Autodesk Inventor part; units mm, degrees
ref_plane "YZ Plane" through (0, 0, 0) normal (1, 0, 0) x (0, 1, 0)
ref_plane "XZ Plane" through (0, 0, 0) normal (0, 1, 0) x (-1, 0, 0)
ref_plane "XY Plane" through (0, 0, 0) normal (0, 0, 1) x (1, 0, 0)
ref_plane "Work Plane1" through (0, -18, -3) normal (1, 0, 0) x (0, 0, -1)
sketch "Sketch2" plane through (0, -18, -3) normal (1, 0, 0) x (0, 0, -1)
  line L0 (-2.3324, 4.2554) -> (0, 4.2554)
  arc A0 (-3, 4) -> (-2.3324, 4.2554) centre (-3, 5) ccw
  line L1 (-3, 0.5) -> (-3, 4)
  line L2 (0, 0.5) -> (-3, 0.5)
  line L3 (0, 4.2554) -> (0, 0.5)
  line L4 (0, 15.7446) -> (-2.3324, 15.7446)
  line L5 (0, 19.5) -> (0, 15.7446)
  line L6 (-3, 19.5) -> (0, 19.5)
  line L7 (-3, 16) -> (-3, 19.5)
  arc A1 (-2.3324, 15.7446) -> (-3, 16) centre (-3, 15) ccw
  line L8 (20, 4.2554) -> (22.3324, 4.2554)
  line L9 (20, 0.5) -> (20, 4.2554)
  line L10 (23, 0.5) -> (20, 0.5)
  line L11 (23, 4) -> (23, 0.5)
  arc A2 (22.3324, 4.2554) -> (23, 4) centre (23, 5) ccw
  line L12 (22.3324, 15.7446) -> (20, 15.7446)
  arc A3 (23, 16) -> (22.3324, 15.7446) centre (23, 15) ccw
  line L13 (23, 19.5) -> (23, 16)
  line L14 (20, 19.5) -> (23, 19.5)
  line L15 (20, 15.7446) -> (20, 19.5)
  line L16 (20, 4.2554) -> (20, 15.7446)
  line L17 (0, 15.7446) -> (0, 4.2554)
  line L18 (20, 10) -> (0, 10)
  line L19 (23, -10) -> (-3, -10)
  line L20 (-3, -10) -> (-3, 30)
  line L21 (-3, 30) -> (23, 30)
  line L22 (23, 30) -> (23, -10)
  line L23 (23, -10) -> (-3, 30) construction
  line L24 (-3, -10) -> (23, 30) construction
  line L25 (26, -16) -> (-6, -16)
  line L26 (-6, -16) -> (-6, 36)
  line L27 (-6, 36) -> (26, 36)
  line L28 (26, 36) -> (26, -16)
  line L29 (26, -16) -> (-6, 36) construction
  line L30 (-6, -16) -> (26, 36) construction
  point P0 (-3, 18)
  point P1 (10, 10)
  point P2 (-3, 4)
  dimension "d2" = 26
  dimension "d3" = 40
  dimension "d4" = 6
  dimension "d5" = 3
extrude "Extrusion1" add sketch "Sketch2" along normal mid plane 4
ref_plane "Work Plane2" through (-2, -34, -13) normal (0, 0, 1) x (1, 0, 0)
sketch "Sketch3" plane through (-2, -34, 3) normal (0, 0, 1) x (1, 0, 0)
  circle A0 centre (2, 26) radius 1.5
  line L0 (0, 0) -> (4, 0)
  line L1 (4, 52) -> (4, 0)
  line L2 (0, 52) -> (4, 52)
  line L3 (0, 0) -> (0, 52)
  line L4 (7, 20) -> (-3, 20)
  line L5 (-3, 20) -> (-3, 32)
  line L6 (-3, 32) -> (7, 32)
  line L7 (7, 32) -> (7, 20)
  line L8 (7, 20) -> (-3, 32) construction
  line L9 (-3, 20) -> (7, 32) construction
  point P0 (2, 34)
  point P1 (0, 20)
  point P2 (0, 32)
  dimension "d8" = 10
  dimension "d9" = 12
extrude "Extrusion2" add sketch "Sketch3" against normal up to surface (3 mm away) contours L4 L5 L6 L3
sketch "Sketch4" plane through (-2, -34, 3) normal (0, 0, 1) x (1, 0, 0)
  circle A0 centre (2, 18) radius 0.7
  circle A1 centre (2, 34) radius 0.7
  circle A2 centre (2, 26) radius 1.5
  line L0 (2, 26) -> (6, 26) construction
  line L1 (2, 24) -> (6, 24)
  line L2 (6, 28) -> (2, 28)
  arc A3 (2, 28) -> (2, 24) centre (2, 26) ccw
  arc A4 (6, 24) -> (6, 28) centre (6, 26) ccw
  point P0 (4, 26)
  dimension "d12" = 4
  dimension "d13" = 4
extrude "Extrusion3" cut sketch "Sketch4" against normal blind 4 contours A0 | A1 | A2 | A3 L2 A4 L1
mirror "Mirror1" about plane through (-2, -34, -13) normal (0, 0, 1) of "Extrusion3", "Extrusion2"
sketch "Sketch5" plane through (-2, -18, -3) normal (-1, 0, 0) x (0, 0, 1)
  line L0 (-26, 16) -> (-23, 16)
  line L1 (-23, 16) -> (-23, 30)
  line L2 (-23, 30) -> (3, 30)
  line L3 (3, 30) -> (3, 16)
  line L4 (3, 16) -> (6, 16)
  line L5 (6, 16) -> (6, 36)
  line L6 (6, 36) -> (-26, 36)
  line L7 (-26, 36) -> (-26, 16)
  line L8 (3, 16) -> (3, 4)
  line L9 (-23, 16) -> (-23, 4)
  line L10 (3, 10) -> (-23, 10)
  line L11 (-2.5, -13) -> (-17.5, -13)
  line L12 (-17.5, -13) -> (-17.5, 33)
  line L13 (-17.5, 33) -> (-2.5, 33)
  line L14 (-2.5, 33) -> (-2.5, -13)
  line L15 (-2.5, -13) -> (-17.5, 33) construction
  line L16 (-17.5, -13) -> (-2.5, 33) construction
  line L17 (-23, 30) -> (3, 30)
  circle A0 centre (-2.5, 33) radius 1
  circle A1 centre (-17.5, 33) radius 1
  point P0 (3, 18)
  point P1 (-10, 10)
  dimension "d16" = 15
  dimension "d17" = 46
  dimension "d18" = 2
  dimension "d19" = 2
extrude "Extrusion4" cut sketch "Sketch5" against normal blind 4 contours A1 L13 L12 | L12 L13 A1 | A0 L13 L14 | L14 L13 A0
ref_plane "Work Plane3" through (-2, -8, 3) normal (0, 1, 0) x (1, 0, 0)
mirror "Mirror2" about plane through (-2, -8, 3) normal (0, 1, 0) of "Extrusion4"
properties part number "cpr_shell_1"
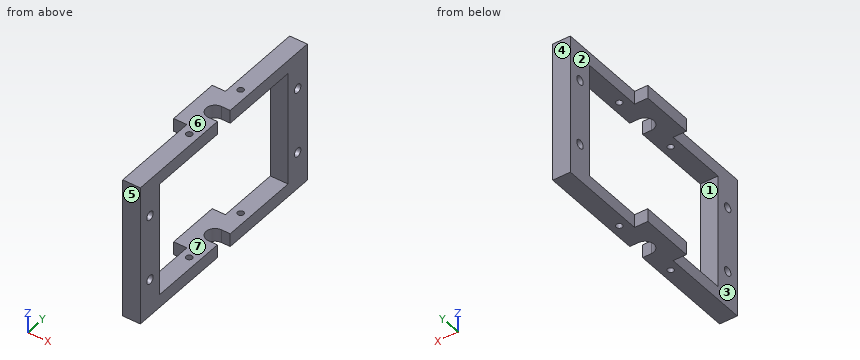
The model under review builds one solid part; all positions refer to its coordinate system, in mm. Face numbers are marked on the shaded views. A direction names the side the tool comes from. Round coordinates to 2 decimals unless told otherwise and drop trailing zeros. Loops run counter-clockwise (first coordinate to the right, second up) from the corner with the lowest first, then second, coordinate; pieces in that order, holes last. Notation, with made-up numbers: M 45.25,21 L 58.25,21 A16 cw 58.25,38 Z; hole C 61,2.25 d10. An arc over 180 degrees is marked long. Answer as a JSON object with one key per item and string values.
(1) To check wall thickness, follow line 1 along Y through (x, z) = (0, 2.2); line 2 along Z through (x, y) = (-0.2, 15); line 3 along Y through (x, z) = (-1.1, -5.5). State the ranges of each line that lie inside material, in increasing order.
Resolved:
{"line 1": "-34 to -16.7, -15.3 to -10, -6 to -0.7, 0.7 to 18", "line 2": "-29 to -21.5, -19.5 to -6.5, -4.5 to 3", "line 3": "-34 to -32, -30 to -28, 12 to 14, 16 to 18"}
(2) Take a section at B-B on z = -25. Give the boundary of the cut face in (x, y).
Resolved:
{"outline": "M -2,-34 L 2,-34 L 2,-28 L -2,-28 Z; M -2,12 L 2,12 L 2,18 L -2,18 Z"}
(3) Draft analysis for pull direction Y (two halves, no side actions). For the marked faces 4, 5, 6 and 7, state which applies: released by +Y, released by -Y, zero draft, split by the parting line, or undercut.
Resolved:
{"face 4": "released by +Y", "face 5": "released by -Y", "face 6": "zero draft", "face 7": "undercut"}
(4) Tool access review of the marked faces 1, 2 and 3: name each direction out of +Z, -Z, +X, -X, +Y, -Y from which nothing blocks a thin tool from reaching the whole face with its end or side.
Resolved:
{"face 1": "+X, -X", "face 2": "+Z, -Z, -X, +Y", "face 3": "+Z, -Z, -X, -Y"}
(5) Take a section at A-A on y = 0. Give the boundary of the cut face in (x, z), and give its area (3 significant figures).
Resolved:
{"outline": "M -2,-29 L -0.7,-29 L -0.7,-26 L -2,-26 Z; M -2,0 L -0.7,0 L -0.7,3 L -2,3 Z; M 0.7,-29 L 2,-29 L 2,-26 L 0.7,-26 Z; M 0.7,0 L 2,0 L 2,3 L 0.7,3 Z", "area": "15.6 mm²"}
(6) Take a section at C-C on x = -3.25. Give the boundary of the cut face in (y, z).
Resolved:
{"outline": "M -14,-29 L -2,-29 L -2,-26 L -14,-26 Z; M -14,0 L -2,0 L -2,3 L -14,3 Z"}
(7) Take a section at D-D on y = -31. Give the boundary of the cut face in (x, z).
Resolved:
{"outline": "M -2,-29 L 2,-29 L 2,-21.5 L -2,-21.5 Z; M -2,-19.5 L 2,-19.5 L 2,-6.5 L -2,-6.5 Z; M -2,-4.5 L 2,-4.5 L 2,3 L -2,3 Z"}
(8) Clearance check with flat-ended pins moving along their axes: P1, Ø3, axis at y = 15, z = -20.5, coming from the -X side; P2, Ø3, axis at y = -31, z = -5.5, coming from the +X side; P3, Ø2.5, axis at x = -3.5, z = -27.5, coming from the -Y side; P4, Ø1.5, axis at x = -4, z = -28, coming from the +Y side. State where each tip first meets the part, or that it passes through.
Resolved:
{"P1": "x = -2", "P2": "x = 2", "P3": "y = -14", "P4": "y = -2"}
